from build123d import *

# Parameters (mm, degrees)
EXTRUDE1_DEPTH              = 25.4
F_1_4_20_TAPPED_HOLE1_D     = 5.1054
F_1_4_20_TAPPED_HOLE1_DEPTH = 16.002
F_1_4_20_TAPPED_HOLE1_TIP   = 1.533816902
F_1_4_20_TAPPED_HOLE2_D     = 5.1054
F_1_4_20_TAPPED_HOLE2_DEPTH = 16.002
F_1_4_20_TAPPED_HOLE2_TIP   = 1.533816902


with BuildPart() as part:
    # Sketch1 → Extrude1 (new body)
    with BuildSketch(Plane.XY):
        Polygon((-6.35, 51.987941466), (6.35, 68.580838747), (6.35, -71.008376889), (-6.35, -71.008376889), align=None)
    extrude(amount=EXTRUDE1_DEPTH)

    # 1/4-20 Tapped Hole1
    with Locations(Plane(origin=(-36.866449815, 12.117365312, 18.061260674), x_dir=(0.6077917109691768, 0.7940964904072809, 0), z_dir=(-0.7940964904072809, 0.6077917109691768, 0))):
        with Locations((59.446155795, 5.361260674)):
            Hole(F_1_4_20_TAPPED_HOLE1_D / 2, depth=F_1_4_20_TAPPED_HOLE1_DEPTH)
            with Locations((0, 0, -(F_1_4_20_TAPPED_HOLE1_DEPTH + F_1_4_20_TAPPED_HOLE1_TIP / 2))):  # 118° drill point
                Cone(0, F_1_4_20_TAPPED_HOLE1_D / 2, F_1_4_20_TAPPED_HOLE1_TIP, mode=Mode.SUBTRACT)

    # 1/4-20 Tapped Hole2
    with Locations(Plane(origin=(-43.242259668, -71.008376889, 18.061260674), x_dir=(-1, 0, 0), z_dir=(0, -1, 0))):
        with Locations((-43.110887349, 5.361260674)):
            Hole(F_1_4_20_TAPPED_HOLE2_D / 2, depth=F_1_4_20_TAPPED_HOLE2_DEPTH)
            with Locations((0, 0, -(F_1_4_20_TAPPED_HOLE2_DEPTH + F_1_4_20_TAPPED_HOLE2_TIP / 2))):  # 118° drill point
                Cone(0, F_1_4_20_TAPPED_HOLE2_D / 2, F_1_4_20_TAPPED_HOLE2_TIP, mode=Mode.SUBTRACT)


solid = part.part
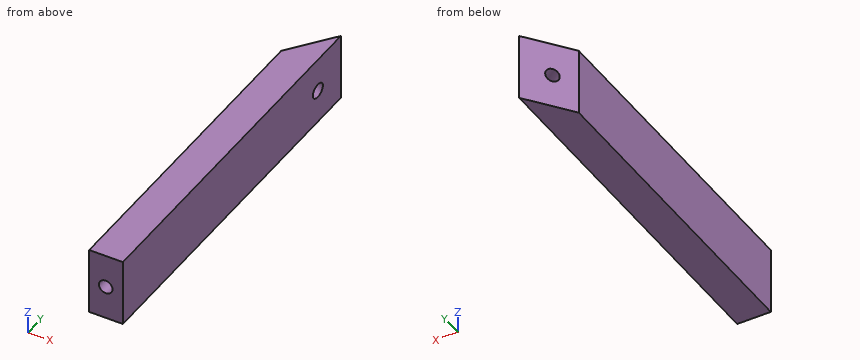
Part model, mm, in its own coordinate system. Coordinates: 2 decimals unless noted, no trailing zeros. Loops run counter-clockwise (first coordinate to the right, second up) from the corner with the lowest first, then second, coordinate; pieces in that order, holes last. Notation, with made-up numbers: (69.5, 66.5) -> (100.5, 66.5) arc R24 cw to (100.5, 101.5) -> close; hole circle Ø7 at (-11, 58). An arc over 180 degrees is marked (long way). Use a Markdown table: item, result. Add a question column.
Item 1: Band-saw the part on A-A on z = 7. Write the cut outline in (x, y).
Item 2: Flat gauge pin, fed straight in: P1, Ø4, axis at x = -0.13, z = 12.7, coming from the +Y side. Where does the tip first touch, or does it go through?
Item 3: Probe probe 1 along X at (y, z) = (-58.25, 12.7); probe 2 along Y at (x, z) = (-3, 18); probe 3 along Y at (x, z) = (3, 20.5). List the from-to ranges inside material, lowest first.
Geometry says:
| question | item | result |
|---|---|---|
| 1 | outline | (-6.35, -71.01) -> (6.35, -71.01) -> (6.35, 68.58) -> (-6.35, 51.99) -> close |
| 2 | P1 | y = 62.73 |
| 3 | probe 1 | -6.35 to -2.68, 2.42 to 6.35 |
| 3 | probe 2 | -71.01 to 56.36 |
| 3 | probe 3 | -71.01 to 64.2 |
